from build123d import *

# Parameters (mm, degrees)
CUT_EXTRUDE1_START = -14
SKETCH2_R          = 2
CUT_EXTRUDE1_DEPTH = 14


with BuildPart() as part:
    # Sketch1 → Revolve1 (revolve)
    with BuildSketch(Plane.XY, mode=Mode.PRIVATE) as revolve1_sk:
        Polygon((0, 0), (0, 2.5), (106, 2.5), (106, 2), (112.5, 2), (112.5, 0), align=None)
    revolve(revolve1_sk.sketch.rotate(Axis((0, 0, 0), (1, 0, 0)), 90), axis=Axis((0, 0, 0), (1, 0, 0)))

    # Sketch2 → Cut-Extrude1 (cut)
    with BuildSketch(Plane.ZY.offset(CUT_EXTRUDE1_START)):
        Circle(SKETCH2_R)
    extrude(amount=CUT_EXTRUDE1_DEPTH, mode=Mode.SUBTRACT)


solid = part.part
Input: part model. Units: mm. Frame: model coordinates. A direction names the side the tool comes from. Give positions to 0.01 mm unless a question says otherwise; leave off trailing zeros. Write each loop counter-clockwise with the first axis right and the second up, starting at its lowest first coordinate (ties: lowest second). Pieces come first, ordered by that corner, then holes. Notation, with made-up numbers: M 62.5,-11 L 78.5,-11 A30 ccw 78.5,13 Z; hole C 58,8.25 d10. An arc over 180 degrees is marked long. Write item = value, one per line. Start each with the question number.
1) Cut plane A-A on z = 0. Return the cut outline in (x, y).
2) Reachability of faces 4 (the flat face through (14, 0, 0)), 5 (the cylindrical face through (53.7, -0.1, -2.5)) from +Z, -Z, +X, -X, +Y, -Y: full face, straight path, thin tool, end or side. Return the list, or none.
3) Cut plane C-C on x = 12. Return the cut outline in (y, z), then the cut area to 3 significant figures.
4) Material intervals for line 1 along Y through (x, z) = (10, 0); line 2 along X through (y, z) = (-2.1, 0.1); line 3 along X through (y, z) = (-1.15, 0.05), sorted ascending. Write a range as [from, to].
5) Cut plane D-D on x = 49.5. Return the cut outline in (y, z).
6) First-contact query: pin 1 Ø1.2 at (y, z) = (-0.5, 0) entering from -X; pin 2 Ø2 at (x, z) = (23.5, -1.5) entering from +Y; pin 3 Ø2 at (x, y) = (37, -2) entering from -Z; pin 4 Ø1.5 at (y, z) = (1, -1.5) entering from -X. Flat tips, straight axial feed; report the tip coordinate or a pass-through.
7) Draft query along Y for faces 1 (the cylindrical face through (109, 2, 0)), 2 (the flat face through (106, -2, -1)), 3 (the cylindrical face through (7, -2, 0)). Return one class per face: +Y half, -Y half, draft (parallel to the pull), parting line (faces both ways), or undercut.
Solved:
q1.outline = M 0,-2.5 L 106,-2.5 L 106,-2 L 112.5,-2 L 112.5,2 L 106,2 L 106,2.5 L 0,2.5 L 0,2 L 14,2 L 14,-2 L 0,-2 Z
q2.face_4 = -X
q2.face_5 = +X, -X
q3.outline = C 0,0 d5; hole C 0,0 d4
q3.area = 7.07 mm2
q4.line_1 = [-2.5, -2], [2, 2.5]
q4.line_2 = [0, 106]
q4.line_3 = [14, 112.5]
q5.outline = C 0,0 d5
q6.pin_1 = 14
q6.pin_2 = 2.45
q6.pin_3 = -2.29
q6.pin_4 = 0
q7.face_1 = parting line
q7.face_2 = draft
q7.face_3 = undercut
